from build123d import *

# Parameters (mm, degrees)
SALIENTE_EXTRUIR1_DEPTH = 15
CROQUIS3_R              = 18
SALIENTE_EXTRUIR2_DEPTH = 0.5
CROQUIS4_R              = 3.5
CORTAR_EXTRUIR1_DEPTH   = 24.5
CROQUIS5_R              = 10
CORTAR_EXTRUIR2_DEPTH   = 0.5
CORTAR_EXTRUIR3_START   = -0.3
CROQUIS6_R              = 26.676513241
CROQUIS6_R_2            = 18
CORTAR_EXTRUIR3_DEPTH   = 0.3


with BuildPart() as part:
    # Croquis2 → Saliente-Extruir1 (new body)
    with BuildSketch(Plane(origin=(0, 0, 0), x_dir=(1, 0, 0), z_dir=(0, 1, 0))):
        with BuildLine():
            Line((-1.253633745, 27.971921679), (-1.253633745, 29.973795262))
            Line((-1.253633745, 29.973795262), (1.253633745, 29.973795262))
            Line((1.253633745, 29.973795262), (1.253633745, 27.971921679))
            ThreePointArc((1.253633745, 27.971921679), (2.926796971, 27.84661307), (4.589450692, 27.62131319))
            Line((4.589450692, 27.62131319), (5.005663613, 29.579441032))
            Line((5.005663613, 29.579441032), (7.458141293, 29.058150809))
            Line((7.458141293, 29.058150809), (7.041928372, 27.100022967))
            ThreePointArc((7.041928372, 27.100022967), (8.652475842, 26.629582456), (10.231954111, 26.063520773))
            Line((10.231954111, 26.063520773), (11.046189452, 27.892323292))
            Line((11.046189452, 27.892323292), (13.336692279, 26.872525729))
            Line((13.336692279, 26.872525729), (12.522456938, 25.04372321))
            ThreePointArc((12.522456938, 25.04372321), (14, 24.248711306), (15.427272037, 23.366627431))
            Line((15.427272037, 23.366627431), (16.603943806, 24.98617718))
            Line((16.603943806, 24.98617718), (18.632365815, 23.512442326))
            Line((18.632365815, 23.512442326), (17.455694046, 21.892892577))
            ThreePointArc((17.455694046, 21.892892577), (18.735656978, 20.808055113), (19.948344146, 19.648500345))
            Line((19.948344146, 19.648500345), (21.436026141, 20.98801523))
            Line((21.436026141, 20.98801523), (23.113715557, 19.124752368))
            Line((23.113715557, 19.124752368), (21.626033563, 17.785237483))
            ThreePointArc((21.626033563, 17.785237483), (22.652475842, 16.457987064), (23.597577894, 15.07163951))
            Line((23.597577894, 15.07163951), (25.331251272, 16.072576302))
            Line((25.331251272, 16.072576302), (26.584885018, 13.901218961))
            Line((26.584885018, 13.901218961), (24.85121164, 12.900282169))
            ThreePointArc((24.85121164, 12.900282169), (25.579272814, 11.388626006), (26.215484254, 9.836075707))
            Line((26.215484254, 9.836075707), (28.11937917, 10.454688665))
            Line((28.11937917, 10.454688665), (28.894167434, 8.070135579))
            Line((28.894167434, 8.070135579), (26.990272518, 7.451522622))
            ThreePointArc((26.990272518, 7.451522622), (27.388132821, 5.821527343), (27.687648157, 4.170628196))
            Line((27.687648157, 4.170628196), (29.678555267, 4.379880966))
            Line((29.678555267, 4.379880966), (29.940636085, 1.886348549))
            Line((29.940636085, 1.886348549), (27.949728974, 1.677095779))
            ThreePointArc((27.949728974, 1.677095779), (28, 0), (27.949728974, -1.677095779))
            Line((27.949728974, -1.677095779), (29.940636085, -1.886348549))
            Line((29.940636085, -1.886348549), (29.678555267, -4.379880966))
            Line((29.678555267, -4.379880966), (27.687648157, -4.170628196))
            ThreePointArc((27.687648157, -4.170628196), (27.388132821, -5.821527343), (26.990272518, -7.451522622))
            Line((26.990272518, -7.451522622), (28.894167434, -8.070135579))
            Line((28.894167434, -8.070135579), (28.11937917, -10.454688665))
            Line((28.11937917, -10.454688665), (26.215484254, -9.836075707))
            ThreePointArc((26.215484254, -9.836075707), (25.579272814, -11.388626006), (24.85121164, -12.900282169))
            Line((24.85121164, -12.900282169), (26.584885018, -13.901218961))
            Line((26.584885018, -13.901218961), (25.331251272, -16.072576302))
            Line((25.331251272, -16.072576302), (23.597577894, -15.07163951))
            ThreePointArc((23.597577894, -15.07163951), (22.652475842, -16.457987064), (21.626033563, -17.785237483))
            Line((21.626033563, -17.785237483), (23.113715557, -19.124752368))
            Line((23.113715557, -19.124752368), (21.436026141, -20.98801523))
            Line((21.436026141, -20.98801523), (19.948344146, -19.648500345))
            ThreePointArc((19.948344146, -19.648500345), (18.735656978, -20.808055113), (17.455694046, -21.892892577))
            Line((17.455694046, -21.892892577), (18.632365815, -23.512442326))
            Line((18.632365815, -23.512442326), (16.603943806, -24.98617718))
            Line((16.603943806, -24.98617718), (15.427272037, -23.366627431))
            ThreePointArc((15.427272037, -23.366627431), (14, -24.248711306), (12.522456938, -25.04372321))
            Line((12.522456938, -25.04372321), (13.336692279, -26.872525729))
            Line((13.336692279, -26.872525729), (11.046189452, -27.892323292))
            Line((11.046189452, -27.892323292), (10.231954111, -26.063520773))
            ThreePointArc((10.231954111, -26.063520773), (8.652475842, -26.629582456), (7.041928372, -27.100022967))
            Line((7.041928372, -27.100022967), (7.458141293, -29.058150809))
            Line((7.458141293, -29.058150809), (5.005663613, -29.579441032))
            Line((5.005663613, -29.579441032), (4.589450692, -27.62131319))
            ThreePointArc((4.589450692, -27.62131319), (2.926796971, -27.84661307), (1.253633745, -27.971921679))
            Line((1.253633745, -27.971921679), (1.253633745, -29.973795262))
            Line((1.253633745, -29.973795262), (-1.253633745, -29.973795262))
            Line((-1.253633745, -29.973795262), (-1.253633745, -27.971921679))
            ThreePointArc((-1.253633745, -27.971921679), (-2.926796971, -27.84661307), (-4.589450692, -27.62131319))
            Line((-4.589450692, -27.62131319), (-5.005663613, -29.579441032))
            Line((-5.005663613, -29.579441032), (-7.458141293, -29.058150809))
            Line((-7.458141293, -29.058150809), (-7.041928372, -27.100022967))
            ThreePointArc((-7.041928372, -27.100022967), (-8.652475842, -26.629582456), (-10.231954111, -26.063520773))
            Line((-10.231954111, -26.063520773), (-11.046189452, -27.892323292))
            Line((-11.046189452, -27.892323292), (-13.336692279, -26.872525729))
            Line((-13.336692279, -26.872525729), (-12.522456938, -25.04372321))
            ThreePointArc((-12.522456938, -25.04372321), (-14, -24.248711306), (-15.427272037, -23.366627431))
            Line((-15.427272037, -23.366627431), (-16.603943806, -24.98617718))
            Line((-16.603943806, -24.98617718), (-18.632365815, -23.512442326))
            Line((-18.632365815, -23.512442326), (-17.455694046, -21.892892577))
            ThreePointArc((-17.455694046, -21.892892577), (-18.735656978, -20.808055113), (-19.948344146, -19.648500345))
            Line((-19.948344146, -19.648500345), (-21.436026141, -20.98801523))
            Line((-21.436026141, -20.98801523), (-23.113715557, -19.124752368))
            Line((-23.113715557, -19.124752368), (-21.626033563, -17.785237483))
            ThreePointArc((-21.626033563, -17.785237483), (-22.652475842, -16.457987064), (-23.597577894, -15.07163951))
            Line((-23.597577894, -15.07163951), (-25.331251272, -16.072576302))
            Line((-25.331251272, -16.072576302), (-26.584885018, -13.901218961))
            Line((-26.584885018, -13.901218961), (-24.85121164, -12.900282169))
            ThreePointArc((-24.85121164, -12.900282169), (-25.579272814, -11.388626006), (-26.215484254, -9.836075707))
            Line((-26.215484254, -9.836075707), (-28.11937917, -10.454688665))
            Line((-28.11937917, -10.454688665), (-28.894167434, -8.070135579))
            Line((-28.894167434, -8.070135579), (-26.990272518, -7.451522622))
            ThreePointArc((-26.990272518, -7.451522622), (-27.388132821, -5.821527343), (-27.687648157, -4.170628196))
            Line((-27.687648157, -4.170628196), (-29.678555267, -4.379880966))
            Line((-29.678555267, -4.379880966), (-29.940636085, -1.886348549))
            Line((-29.940636085, -1.886348549), (-27.949728974, -1.677095779))
            ThreePointArc((-27.949728974, -1.677095779), (-28, 0), (-27.949728974, 1.677095779))
            Line((-27.949728974, 1.677095779), (-29.940636085, 1.886348549))
            Line((-29.940636085, 1.886348549), (-29.678555267, 4.379880966))
            Line((-29.678555267, 4.379880966), (-27.687648157, 4.170628196))
            ThreePointArc((-27.687648157, 4.170628196), (-27.388132821, 5.821527343), (-26.990272518, 7.451522622))
            Line((-26.990272518, 7.451522622), (-28.894167434, 8.070135579))
            Line((-28.894167434, 8.070135579), (-28.11937917, 10.454688665))
            Line((-28.11937917, 10.454688665), (-26.215484254, 9.836075707))
            ThreePointArc((-26.215484254, 9.836075707), (-25.579272814, 11.388626006), (-24.85121164, 12.900282169))
            Line((-24.85121164, 12.900282169), (-26.584885018, 13.901218961))
            Line((-26.584885018, 13.901218961), (-25.331251272, 16.072576302))
            Line((-25.331251272, 16.072576302), (-23.597577894, 15.07163951))
            ThreePointArc((-23.597577894, 15.07163951), (-22.652475842, 16.457987064), (-21.626033563, 17.785237483))
            Line((-21.626033563, 17.785237483), (-23.113715557, 19.124752368))
            Line((-23.113715557, 19.124752368), (-21.436026141, 20.98801523))
            Line((-21.436026141, 20.98801523), (-19.948344146, 19.648500345))
            ThreePointArc((-19.948344146, 19.648500345), (-18.735656978, 20.808055113), (-17.455694046, 21.892892577))
            Line((-17.455694046, 21.892892577), (-18.632365815, 23.512442326))
            Line((-18.632365815, 23.512442326), (-16.603943806, 24.98617718))
            Line((-16.603943806, 24.98617718), (-15.427272037, 23.366627431))
            ThreePointArc((-15.427272037, 23.366627431), (-14, 24.248711306), (-12.522456938, 25.04372321))
            Line((-12.522456938, 25.04372321), (-13.336692279, 26.872525729))
            Line((-13.336692279, 26.872525729), (-11.046189452, 27.892323292))
            Line((-11.046189452, 27.892323292), (-10.231954111, 26.063520773))
            ThreePointArc((-10.231954111, 26.063520773), (-8.652475842, 26.629582456), (-7.041928372, 27.100022967))
            Line((-7.041928372, 27.100022967), (-7.458141293, 29.058150809))
            Line((-7.458141293, 29.058150809), (-5.005663613, 29.579441032))
            Line((-5.005663613, 29.579441032), (-4.589450692, 27.62131319))
            ThreePointArc((-4.589450692, 27.62131319), (-2.926796971, 27.84661307), (-1.253633745, 27.971921679))
        make_face()
    extrude(amount=SALIENTE_EXTRUIR1_DEPTH)

    # Croquis3 → Saliente-Extruir2 (add)
    with BuildSketch(Plane.XZ):
        with Locations(Location((0, 0, 0), (0, 0, 90))):
            Circle(CROQUIS3_R)
    extrude(amount=SALIENTE_EXTRUIR2_DEPTH)

    # Croquis4 → Cortar-Extruir1 (cut)
    with BuildSketch(Plane.XZ.offset(0.5)):
        with Locations(Location((0, 0, 0), (0, 0, 270))):
            Circle(CROQUIS4_R)
    extrude(amount=-CORTAR_EXTRUIR1_DEPTH, mode=Mode.SUBTRACT)

    # Croquis5 → Cortar-Extruir2 (cut)
    with BuildSketch(Plane(origin=(0, -0.5, 0), x_dir=(-1, 0, 0), z_dir=(0, -1, 0))):
        with Locations(Location((0, 0, 0), (0, 0, 90))):
            Circle(CROQUIS5_R)
    extrude(amount=-CORTAR_EXTRUIR2_DEPTH, mode=Mode.SUBTRACT)

    # Croquis6 → Cortar-Extruir3 (cut)
    with BuildSketch(Plane.XZ.offset(CORTAR_EXTRUIR3_START)):
        with Locations(Location((0, 0, 0), (0, 0, 270))):
            Circle(CROQUIS6_R)
        with Locations(Location((0, 0, 0), (0, 0, 270))):
            Circle(CROQUIS6_R_2, mode=Mode.SUBTRACT)
    extrude(amount=CORTAR_EXTRUIR3_DEPTH, mode=Mode.SUBTRACT)


solid = part.part
Design review of the part built by this model. Coordinates are the model's own, in mm. A direction names the side the tool comes from. Coordinates: 2 decimals unless noted, no trailing zeros. Loops run counter-clockwise (first coordinate to the right, second up) from the corner with the lowest first, then second, coordinate; pieces in that order, holes last. Notation, with made-up numbers: M 75.5,7 L 92.5,7 A25 cw 92.5,23 Z; hole C -24,12 d9. An arc over 180 degrees is marked long. Use one line per item in the form item = value.
(1) Consider section C-C (z = -9). Write out the cut boundary in (x, y), and give its area (3 significant figures).
Return value:
outline = M -28.59,0 L -25.11,0 L -25.11,0.3 L -15.59,0.3 L -15.59,-0.5 L -4.36,-0.5 L -4.36,0 L 4.36,0 L 4.36,-0.5 L 15.59,-0.5 L 15.59,0.3 L 25.11,0.3 L 25.11,0 L 28.59,0 L 28.59,15 L -28.59,15 Z
area = 863 mm2
(2) Draft analysis for pull direction Z (two halves, no side actions). For faces 6 (the face through (-29.81, 7.4, -3.12)), 7 (the face through (-1.254, 7, 29)), 8 (the face through (-28, 7, 0)), state which applies: pulls with the +Z half, pulls with the -Z half, needs draft (parallel to the pull), parting line crosses it, or undercut.
Return value:
face_6 = pulls with the -Z half
face_7 = needs draft
face_8 = undercut
(3) Consider section D-D (x = -14.5). Write out the cut boundary in (y, z).
Return value:
outline = M -0.5,-10.67 L 0.3,-10.67 L 0.3,-22.39 L 0,-22.39 L 0,-23.95 L 15,-23.95 L 15,23.95 L 0,23.95 L 0,22.39 L 0.3,22.39 L 0.3,10.67 L -0.5,10.67 Z
(4) Consider section B-B (z = 0). Write out the cut boundary in (x, y), and give its area (3 significant figures).
Return value:
outline = M -28,0 L -26.68,0 L -26.68,0.3 L -18,0.3 L -18,-0.5 L -10,-0.5 L -10,0 L -3.5,0 L -3.5,15 L -28,15 Z; M 3.5,0 L 10,0 L 10,-0.5 L 18,-0.5 L 18,0.3 L 26.68,0.3 L 26.68,0 L 28,0 L 28,15 L 3.5,15 Z
area = 738 mm2
(5) Consider section A-A (x = 0). Write out the cut boundary in (y, z).
Return value:
outline = M -0.5,-18 L 0.3,-18 L 0.3,-26.68 L 0,-26.68 L 0,-29.97 L 15,-29.97 L 15,-3.5 L 0,-3.5 L 0,-10 L -0.5,-10 Z; M -0.5,10 L 0,10 L 0,3.5 L 15,3.5 L 15,29.97 L 0,29.97 L 0,26.68 L 0.3,26.68 L 0.3,18 L -0.5,18 Z
(6) For faces 1 (the face through (0, 7, -29.974)), 2 (the face through (-22.38, 7.395, 18.464)), 3 (the face through (-2.95, 7.395, -27.844)), 4 (the face through (-18.72, 7.4, 20.82)), 5 (the face through (18.05, 7.4, -22.71)), list the 3-axis set-ups (+Z, -Z, +X, -X, +Y, -Y) from which the entire face can be reached by the end or side of a thin tool; tool diameter is ignored.
Return value:
face_1 = -Z, +X, -X, +Y, -Y
face_2 = -X, +Y, -Y
face_3 = -Z, +Y, -Y
face_4 = +Y, -Y
face_5 = +X, +Y, -Y
(7) Clearance check with flat-ended pins moving along their axes: P1, Ø16, axis at x = 0, z = 0, coming from the -Y side; P2, Ø1, axis at y = 10.5, z = -29, coming from the +X side; P3, Ø6, axis at y = 8, z = 7, coming from the -X side. State where each tip first meets the part, or that it passes through.
Return value:
P1 = 0
P2 = 7.46
P3 = -29.72
(8) For line 1 along X through (y, z) = (-0.2, 0); line 2 along Y through (x, z) = (-1.5, -23.5); line 3 along Y through (x, z) = (5, -4), list the stretches that pass through material, from the lowest coordinate up. Write a range as from..to.
Return value:
line_1 = -18..-10, 10..18
line_2 = 0.3..15
line_3 = 0..15
